Autodesk Inventor part; units mm, degrees
ref_plane "1_XY" through (2, 0, 0) normal (1, 0, 0) x (0, 0, -1)
ref_plane "1_YZ" through (2, 0, 0) normal (0, 0, -1) x (0, 1, 0)
ref_plane "1_ZX" through (2, 0, 0) normal (0, 1, 0) x (1, 0, 0)
sketch "Sketch_3" plane through (0, 0, 0) normal (0, 0, 1) x (1, 0, 0)
  line L0 (3.85, 0) -> (0, 0)
  line L1 (0, 7.65) -> (0, 6.35)
  arc A0 (0, 6.35) -> (0.075, 6.275) centre (0.075, 6.35) ccw
  line L2 (0.075, 6.275) -> (0.605, 6.275)
  line L3 (0.605, 6.275) -> (0.605, 6.1668)
  line L4 (0.605, 6.1668) -> (1.5693, 6.1668)
  arc A1 (2.4307, 6.1668) -> (1.5693, 6.1668) centre (2, 5.5) ccw
  line L5 (2.4307, 6.1668) -> (3.4, 6.1668)
  line L6 (3.4, 6.1668) -> (3.4, 6.275)
  line L7 (3.4, 6.275) -> (3.925, 6.275)
  arc A2 (3.925, 6.275) -> (4, 6.35) centre (3.925, 6.35) ccw
  line L8 (4, 6.35) -> (4, 6.85)
  arc A3 (4, 6.85) -> (3.85, 7) centre (3.85, 6.85) ccw
  line L9 (3.85, 7) -> (0.8, 7)
  line L10 (0.8, 7) -> (0.8, 7.65)
  line L11 (0.8, 7.65) -> (0.65, 7.8)
  line L12 (0.65, 7.8) -> (0.15, 7.8)
  line L13 (0.15, 7.8) -> (0, 7.65)
revolve "Revolution1" add sketch "Sketch_3" angle 360 about axis through (3.85, 0, 0) along (1, 0, 0)
ref_plane "1_XY" through (2, 0, 0) normal (1, 0, 0) x (0, 0, -1)
ref_plane "1_YZ" through (2, 0, 0) normal (0, 0, -1) x (0, 1, 0)
ref_plane "1_ZX" through (2, 0, 0) normal (0, 1, 0) x (1, 0, 0)
properties part number "LF-1480ZZ_or" material "鋼、炭素鋼"
Here's how the part is built. I have some questions about the finished solid (model axes, mm). A direction names the side the tool comes from. Round coordinates to 2 decimals unless told otherwise and drop trailing zeros. Order: outer loops, then holes, each group sorted by start corner. A loop starts at its lowest first (then second) coordinate and runs counter-clockwise, first axis right, second up. Notation, with made-up numbers: (62.5, -38.5) -> (73.5, -38.5) arc R9 cw to (73.5, -32.5) -> close; hole circle Ø5 at (60.25, -29). An arc over 180 degrees is marked (long way). Use a Markdown table: item, result. Add a question column.
(1) For pin 1 Ø7.5 at (y, z) = (0, 0) entering from -X; pin 2 Ø1.5 at (x, z) = (1, 1.5) entering from +Y (3 decimals), each with a flat end and sliding along its axis, tell me the tip position at first contact or that it passes through.
(2) Suppose I cut it at C-C, the plane x = 2. Please give me the cut outline in (y, z).
(3) I need wall thicknesses on line 1 along Z through (x, y) = (1.3, 0); line 2 along Z through (x, y) = (3.6, 0) (3 decimals); line 3 along Y through (x, z) = (2.8, 5.5). Which ranges of each line are inside material? Lowest first, please.
(4) Suppose I cut it at D-D, the plane x = 3.15. Please give me the cut outline in (y, z).
(5) For faces 1 (the face through (2.92, -1.34, -6.02)), 2 (the face through (0.8, 7, -2)), which set-ups out of +Z, -Z, +X, -X, +Y, -Y let a thin tool reach every point of the face, with its end or its side?
(6) If we mould it in two halves opening along Y, with no side actions, what happens to faces 3 (the face through (0.3, 5.8, -2.4)), 4 (the face through (0, -3, 6)), 5 (the face through (2.304, 6.466, 2.681)), 6 (the face through (3.7, 5.8, -2.4))? For each: released by +Y, released by -Y, zero draft, split by the parting line, or undercut.
Verdict:
| question | item | result |
|---|---|---|
| 1 | pin 1 | through |
| 1 | pin 2 | y = 7.755 |
| 2 | outline | circle Ø14 at (0, 0); hole circle Ø12.59 at (0, 0) |
| 3 | line 1 | -7 to -6.17, 6.17 to 7 |
| 3 | line 2 | -7 to -6.275, 6.275 to 7 |
| 3 | line 3 | -4.33 to -2.79, 2.79 to 4.33 |
| 4 | outline | circle Ø14 at (0, 0); hole circle Ø12.33 at (0, 0) |
| 5 | face 1 | +X, -X |
| 5 | face 2 | +X |
| 6 | face 3 | undercut |
| 6 | face 4 | zero draft |
| 6 | face 5 | split by the parting line |
| 6 | face 6 | undercut |
